from build123d import *

# Parameters (mm, degrees)
SKETCH1_R           = 2.75
BOSS_EXTRUDE1_DEPTH = 10
SKETCH2_R           = 14.5
CUT_EXTRUDE1_DEPTH  = 2.5
BOSS_EXTRUDE2_DEPTH = 5
CUT_EXTRUDE5_DEPTH  = 41.387552571
SKETCH5_R           = 14.5
CUT_EXTRUDE6_DEPTH  = 2.5


with BuildPart() as part:
    # Sketch1 → Boss-Extrude1 (new, symmetric)
    with BuildSketch(Plane.XY):
        with BuildLine():
            Line((-10.101695673, 3.676716541), (-16.899464568, -15))
            Line((-16.899464568, -15), (16.899464568, -15))
            Line((16.899464568, -15), (10.101695673, 3.676716541))
            ThreePointArc((10.101695673, 3.676716541), (0, 10.75), (-10.101695673, 3.676716541))
        make_face()
        Circle(SKETCH1_R, mode=Mode.SUBTRACT)
    extrude(amount=BOSS_EXTRUDE1_DEPTH, both=True)

    # Sketch2 → Cut-Extrude1 (cut, symmetric)
    with BuildSketch(Plane.XY):
        Circle(SKETCH2_R)
    extrude(amount=CUT_EXTRUDE1_DEPTH, both=True, mode=Mode.SUBTRACT)

    # Sketch3 → Boss-Extrude2 (add)
    with BuildSketch(Plane.XZ.offset(15)):
        with BuildLine():
            Line((-16.899464568, 15), (-16.899464568, 10))
            Line((-16.899464568, 10), (16.899464568, 10))
            Line((16.899464568, 10), (16.899464568, 15))
            ThreePointArc((16.899464568, 15), (15.434998474, 18.535533906), (11.899464568, 20))
            Line((11.899464568, 20), (-11.899464568, 20))
            ThreePointArc((-11.899464568, 20), (-15.434998474, 18.535533906), (-16.899464568, 15))
        make_face()
        Polygon((16.899464568, 10), (-16.899464568, 10), (-16.899464568, -10), (16.899464568, -10), (16.899464568, 0), align=None)
        with BuildLine():
            Line((16.899464568, -10), (-16.899464568, -10))
            Line((-16.899464568, -10), (-16.899464568, -15))
            ThreePointArc((-16.899464568, -15), (-15.434998474, -18.535533906), (-11.899464568, -20))
            Line((-11.899464568, -20), (11.899464568, -20))
            ThreePointArc((11.899464568, -20), (15.434998474, -18.535533906), (16.899464568, -15))
            Line((16.899464568, -15), (16.899464568, -10))
        make_face()
    extrude(amount=BOSS_EXTRUDE2_DEPTH)

    # Sketch4 → Cut-Extrude5 (cut, through all)
    with BuildSketch(Plane.XZ.offset(20)):
        with BuildLine():
            Line((-2.75, 20), (-2.75, 13.75))
            ThreePointArc((-2.75, 13.75), (0, 11), (2.75, 13.75))
            Line((2.75, 13.75), (2.75, 20))
            Line((2.75, 20), (-2.75, 20))
        make_face()
        with BuildLine():
            Line((-2.75, -20), (-2.75, -13.75))
            ThreePointArc((-2.75, -13.75), (0, -11), (2.75, -13.75))
            Line((2.75, -13.75), (2.75, -20))
            Line((2.75, -20), (-2.75, -20))
        make_face()
    extrude(amount=-CUT_EXTRUDE5_DEPTH, mode=Mode.SUBTRACT)

    # Sketch5 → Cut-Extrude6 (cut, symmetric)
    with BuildSketch(Plane.XY):
        Circle(SKETCH5_R)
        with BuildLine():
            ThreePointArc((10.253048327, -10.253048327), (-10.253048327, -10.253048327), (-10.253048327, 10.253048327))
            Line((-10.253048327, 10.253048327), (-31.466251763, -10.960155108))
            Line((-31.466251763, -10.960155108), (-10.960155108, -31.466251763))
            Line((-10.960155108, -31.466251763), (10.253048327, -10.253048327))
        make_face()
    extrude(amount=CUT_EXTRUDE6_DEPTH, both=True, mode=Mode.SUBTRACT)


solid = part.part
Can you work these out from the model? Positions are in its coordinate system, mm. A direction names the side the tool comes from. Give positions to 0.01 mm unless a question says otherwise; leave off trailing zeros. Write each loop counter-clockwise with the first axis right and the second up, starting at its lowest first coordinate (ties: lowest second). Pieces come first, ordered by that corner, then holes. Notation, with made-up numbers: (-36, -27.5) -> (-28, -27.5) arc R28 cw to (-28, 5.5) -> close; hole circle Ø10 at (79.25, 81). An arc over 180 degrees is marked (long way). Answer as a JSON object with one key per item and string values. Group by question number.
Item 1: Suppose I cut it at B-B (z = -16). Please give me the cut outline in (x, y), plus the area to 3 significant figures.
Item 2: We'd pull the mould along Z, two halves only. Please class faces 4 (the face through (0, -5, -10)), 5 (the face through (-2, -4, -2.5)), 6 (the face through (-2.75, -18, -17)): +Z half, -Z half, draft (parallel to the pull), parting line (faces both ways), or undercut.
Item 3: Suppose I cut it at A-A (x = 0). Please give me the cut outline in (y, z), plus the area to 3 significant figures.
Item 4: Suppose I cut it at D-D (z = 6.5). Please give me the cut outline in (x, y), plus the area to 3 significant figures.
Item 5: For faces 1 (the face through (5.311, -15.195, 0.035)), 2 (the face through (-2.75, -18, 17)), 3 (the face through (4, -15, -15)), which set-ups out of +Z, -Z, +X, -X, +Y, -Y let a thin tool reach every point of the face, with its end or its side?
Item 6: Suppose I cut it at C-C (y = 1.5). Please give me the cut outline in (x, z), plus the area to 3 significant figures.
Item 7: I'm going to push flat-ended pins straight in: P1, Ø4, axis at y = -17, z = 18, coming from the -X side; P2, Ø8, axis at x = -13.5, z = -11.5, coming from the +Y side; P3, Ø12, axis at x = 1.5, y = -8.5, coming from the +Z side. Where does each tip first touch, or does it pass through?
Item 8: Please list where these lines run through material, in increasing order: line 1 (Z direction, x = 5.5, y = 5); line 2 (Z direction, x = -6, y = -18); line 3 (X direction, y = -17.5, z = -15). Write a range as [from, to].
Findings:
{
 "1": {"outline": "(-16.8, -20) -> (-2.75, -20) -> (-2.75, -15) -> (-16.8, -15) -> close; (2.75, -20) -> (16.8, -20) -> (16.8, -15) -> (2.75, -15) -> close", "area": "140 mm²"},
 "2": {"face 4": "-Z half", "face 5": "undercut", "face 6": "draft"},
 "3": {"outline": "(-20, -11) -> (-15, -11) -> (-15, -10) -> (-2.75, -10) -> (-2.75, -2.5) -> (-20, -2.5) -> close; (-20, 2.5) -> (-2.75, 2.5) -> (-2.75, 10) -> (-15, 10) -> (-15, 11) -> (-20, 11) -> close; (2.75, -10) -> (10.75, -10) -> (10.75, -2.5) -> (2.75, -2.5) -> close; (2.75, 2.5) -> (10.75, 2.5) -> (10.75, 10) -> (2.75, 10) -> close", "area": "389 mm²"},
 "4": {"outline": "(-16.9, -20) -> (16.9, -20) -> (16.9, -15) -> (10.1, 3.68) arc R10.75 ccw to (-10.1, 3.68) -> (-16.9, -15) -> close; hole circle Ø5.5 at (0, 0)", "area": "754 mm²"},
 "5": {"face 1": "-X, +Y", "face 2": "+Z, +Y, -Y", "face 3": "-Z, +X, -X, +Y"},
 "6": {"outline": "(-10.89, -10) -> (-2.3, -10) -> (-2.3, -2.5) -> (-10.89, -2.5) -> close; (-10.89, 2.5) -> (-2.3, 2.5) -> (-2.3, 10) -> (-10.89, 10) -> close; (2.3, -10) -> (10.89, -10) -> (10.89, -2.5) -> (2.3, -2.5) -> close; (2.3, 2.5) -> (10.89, 2.5) -> (10.89, 10) -> (2.3, 10) -> close", "area": "258 mm²"},
 "7": {"P1": "stops at x = -16.8", "P2": "stops at y = 4.44", "P3": "stops at z = 10"},
 "8": {"line 1": "z = [-10, -2.5], [2.5, 10]", "line 2": "z = [-20, -2.5], [2.5, 20]", "line 3": "x = [-16.9, -2.75], [2.75, 16.9]"}
}
